Geometry: final body of the model. Coordinates: model frame, mm. Give positions to 0.01 mm unless a question says otherwise; leave off trailing zeros. Write each loop counter-clockwise with the first axis right and the second up, starting at its lowest first coordinate (ties: lowest second). Pieces come first, ordered by that corner, then holes.
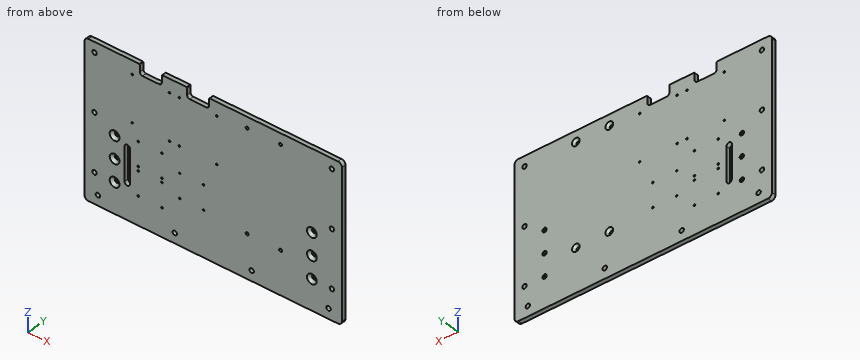
```python
from build123d import *

# Parameters (mm, degrees)
SKETCH1_W                                       = 385
SKETCH1_H                                       = 200
BOSS_EXTRUDE1_DEPTH                             = 6.35
M6_CLEARANCE_HOLE1_D                            = 6.6
CSK_FOR_M6_FLAT_HEAD_MACHINE_SCREW1_AT_2_COUNT  = 2
CSK_FOR_M6_FLAT_HEAD_MACHINE_SCREW1_AT_2_PITCH  = 33
CSK_FOR_M6_FLAT_HEAD_MACHINE_SCREW1_AT_3_COUNT  = 2
CSK_FOR_M6_FLAT_HEAD_MACHINE_SCREW1_AT_3_PITCH  = 66
CSK_FOR_M6_FLAT_HEAD_MACHINE_SCREW1_AT_4_COUNT  = 2
CSK_FOR_M6_FLAT_HEAD_MACHINE_SCREW1_AT_4_PITCH  = 295
CSK_FOR_M6_FLAT_HEAD_MACHINE_SCREW1_AT_5_COUNT  = 2
CSK_FOR_M6_FLAT_HEAD_MACHINE_SCREW1_AT_5_PITCH  = 302.292904316
CSK_FOR_M6_FLAT_HEAD_MACHINE_SCREW1_AT_6_COUNT  = 2
CSK_FOR_M6_FLAT_HEAD_MACHINE_SCREW1_AT_6_PITCH  = 296.840024255
M3X0_5_TAPPED_HOLE1_D                           = 2.5
M3X0_5_TAPPED_HOLE1_DEPTH                       = 7.5
M3X0_5_TAPPED_HOLE1_TIP                         = 0.751075774
CSK_FOR_M4_FLAT_HEAD_MACHINE_SCREW1_D           = 4.5
CSK_FOR_M4_FLAT_HEAD_MACHINE_SCREW1_CSINK_D     = 11.4
CSK_FOR_M4_FLAT_HEAD_MACHINE_SCREW1_CSINK_ANGLE = 90
M3X0_5_TAPPED_HOLE2_D                           = 2.5
CUT_EXTRUDE1_DEPTH                              = 7.35
CUT_EXTRUDE2_DEPTH                              = 7.35
SKETCH18_W                                      = 33
SKETCH18_H                                      = 11
CUT_EXTRUDE3_DEPTH                              = 7.35
FILLET2_R                                       = 1
SKETCH19_W                                      = 385
SKETCH19_H                                      = 6.35
BOSS_EXTRUDE2_DEPTH                             = 30
M6_CLEARANCE_HOLE2_D                            = 6.6
FILLET3_R                                       = 6


with BuildPart() as part:
    # Sketch1 → Boss-Extrude1 (new body)
    with BuildSketch(Plane(origin=(0, 0, 0), x_dir=(1, 0, 0), z_dir=(0, 1, 0))):
        Rectangle(SKETCH1_W, SKETCH1_H)
    extrude(amount=BOSS_EXTRUDE1_DEPTH)

    # M6 Clearance Hole1 (through all)
    with Locations(Plane(origin=(0, 6.35, 0), x_dir=(1, 0, 0), z_dir=(0, 1, 0))):
        with Locations((-177.5, 85), (-177.5, 0), (-177.5, -85)):
            m6_clearance_hole1 = Hole(M6_CLEARANCE_HOLE1_D / 2)

    # Mirror1: M6 Clearance Hole1 across plane
    add(m6_clearance_hole1.mirror(Plane(origin=(0, 0, 0), x_dir=(0, 0, 1), z_dir=(1, 0, 0))), mode=Mode.SUBTRACT)

    # Sketch8 → CSK for M6 Flat Head Machine Screw1 (revolve, cut)
    with BuildSketch(Plane(origin=(147.5, 0, -85), x_dir=(0, 0, -1), z_dir=(1, 0, 0))):
        Polygon((0, 0), (0, 6.35), (3.2, 6.35), (3.2, 4.1), (7.3, 0), align=None)
    csk_for_m6_flat_head_machine_screw1 = revolve(axis=Axis((147.5, -6.35, -85), (0, 1, 0)), mode=Mode.SUBTRACT)

    # CSK for M6 Flat Head Machine Screw1 at 2: CSK for M6 Flat Head Machine Screw1 ×2
    with Locations(*[(0, 0, i * CSK_FOR_M6_FLAT_HEAD_MACHINE_SCREW1_AT_2_PITCH) for i in range(1, CSK_FOR_M6_FLAT_HEAD_MACHINE_SCREW1_AT_2_COUNT)]):
        add(csk_for_m6_flat_head_machine_screw1, mode=Mode.SUBTRACT)

    # CSK for M6 Flat Head Machine Screw1 at 3: CSK for M6 Flat Head Machine Screw1 ×2
    with Locations(*[(0, 0, i * CSK_FOR_M6_FLAT_HEAD_MACHINE_SCREW1_AT_3_PITCH) for i in range(1, CSK_FOR_M6_FLAT_HEAD_MACHINE_SCREW1_AT_3_COUNT)]):
        add(csk_for_m6_flat_head_machine_screw1, mode=Mode.SUBTRACT)

    # CSK for M6 Flat Head Machine Screw1 at 4: CSK for M6 Flat Head Machine Screw1 ×2
    with Locations(*[(-i * CSK_FOR_M6_FLAT_HEAD_MACHINE_SCREW1_AT_4_PITCH, 0, 0) for i in range(1, CSK_FOR_M6_FLAT_HEAD_MACHINE_SCREW1_AT_4_COUNT)]):
        add(csk_for_m6_flat_head_machine_screw1, mode=Mode.SUBTRACT)

    # CSK for M6 Flat Head Machine Screw1 at 5: CSK for M6 Flat Head Machine Screw1 ×2
    with Locations(*[Vector(-0.975874709, 0, 0.218331291) * (i * CSK_FOR_M6_FLAT_HEAD_MACHINE_SCREW1_AT_5_PITCH) for i in range(1, CSK_FOR_M6_FLAT_HEAD_MACHINE_SCREW1_AT_5_COUNT)]):
        add(csk_for_m6_flat_head_machine_screw1, mode=Mode.SUBTRACT)

    # CSK for M6 Flat Head Machine Screw1 at 6: CSK for M6 Flat Head Machine Screw1 ×2
    with Locations(*[Vector(-0.993801293, 0, 0.111170992) * (i * CSK_FOR_M6_FLAT_HEAD_MACHINE_SCREW1_AT_6_PITCH) for i in range(1, CSK_FOR_M6_FLAT_HEAD_MACHINE_SCREW1_AT_6_COUNT)]):
        add(csk_for_m6_flat_head_machine_screw1, mode=Mode.SUBTRACT)

    # M3x0.5 Tapped Hole1
    with Locations(Plane(origin=(0, 0, 0), x_dir=(-1, 0, 0), z_dir=(0, -1, 0))):
        with Locations((-5.317429377, -80), (50.562570623, -80), (65.432985675, -80), (121.312985675, -80), (121.312985675, -11.42), (65.432985675, -11.42), (50.562570623, -11.42), (-5.317429377, -11.42), (76.646256291, 52.44), (76.646256291, 88), (112.206256291, 52.44), (112.206256291, 88), (76.646256291, 46.44), (112.206256291, 46.44), (112.206256291, 10.88), (76.646256291, 10.88)):
            Hole(M3X0_5_TAPPED_HOLE1_D / 2, depth=M3X0_5_TAPPED_HOLE1_DEPTH)
            with Locations((0, 0, -(M3X0_5_TAPPED_HOLE1_DEPTH + M3X0_5_TAPPED_HOLE1_TIP / 2))):  # 118° drill point
                Cone(0, M3X0_5_TAPPED_HOLE1_D / 2, M3X0_5_TAPPED_HOLE1_TIP, mode=Mode.SUBTRACT)

    # CSK for M4 Flat Head Machine Screw1 (through all)
    with Locations(Plane(origin=(0, 6.35, 0), x_dir=(1, 0, 0), z_dir=(0, 1, 0))):
        with Locations((50.75, -84), (100.75, -84), (50.75, 66), (100.75, 66)):
            CounterSinkHole(CSK_FOR_M4_FLAT_HEAD_MACHINE_SCREW1_D / 2, CSK_FOR_M4_FLAT_HEAD_MACHINE_SCREW1_CSINK_D / 2, counter_sink_angle=CSK_FOR_M4_FLAT_HEAD_MACHINE_SCREW1_CSINK_ANGLE)

    # M3x0.5 Tapped Hole2 (through all)
    with Locations(Plane(origin=(0, 0, 0), x_dir=(-1, 0, 0), z_dir=(0, -1, 0))):
        with Locations((14.506651869, 62.535124228), (50.066651869, 62.535124228), (50.066651869, 26.975124228), (14.506651869, 26.975124228)):
            Hole(M3X0_5_TAPPED_HOLE2_D / 2)

    # Sketch16 → Cut-Extrude1 (cut, through all)
    with BuildSketch(Plane.XZ):
        with BuildLine():
            Line((-124.5, -27), (-124.5, -77))
            ThreePointArc((-124.5, -77), (-128.5, -81), (-132.5, -77))
            Line((-132.5, -77), (-132.5, -27))
            ThreePointArc((-132.5, -27), (-128.5, -23), (-124.5, -27))
        make_face()
    extrude(amount=-CUT_EXTRUDE1_DEPTH, mode=Mode.SUBTRACT)

    # Sketch17 → Cut-Extrude2 (cut, through all)
    with BuildSketch(Plane.XZ):
        with BuildLine():
            Line((-105.872985675, 93), (-80.872985675, 93))
            ThreePointArc((-80.872985675, 93), (-76.872985675, 89), (-80.872985675, 85))
            Line((-80.872985675, 85), (-105.872985675, 85))
            ThreePointArc((-105.872985675, 85), (-109.872985675, 89), (-105.872985675, 93))
        make_face()
        with BuildLine():
            Line((-35.122570623, 93), (-10.122570623, 93))
            ThreePointArc((-10.122570623, 93), (-6.122570623, 89), (-10.122570623, 85))
            Line((-10.122570623, 85), (-35.122570623, 85))
            ThreePointArc((-35.122570623, 85), (-39.122570623, 89), (-35.122570623, 93))
        make_face()
    extrude(amount=-CUT_EXTRUDE2_DEPTH, mode=Mode.SUBTRACT)

    # Sketch18 → Cut-Extrude3 (cut, through all)
    with BuildSketch(Plane.XZ):
        with Locations((-22.622570623, 94.5)):
            Rectangle(SKETCH18_W, SKETCH18_H)
        with Locations((-93.372985675, 94.5)):
            Rectangle(SKETCH18_W, SKETCH18_H)
    extrude(amount=-CUT_EXTRUDE3_DEPTH, mode=Mode.SUBTRACT)

    # Fillet2
    fillet2_edges = [part.edges().sort_by_distance(p)[0] for p in [
        (-6.122570623, 3.175, 100),
        (-39.122570623, 3.175, 100),
        (-76.872985675, 3.175, 100),
        (-109.872985675, 3.175, 100),
    ]]
    fillet(fillet2_edges, radius=FILLET2_R)

    # Sketch19 → Boss-Extrude2 (add)
    with BuildSketch(Plane(origin=(0, 0, -100), x_dir=(-1, 0, 0), z_dir=(0, 0, -1))):
        with Locations((0, 3.175)):
            Rectangle(SKETCH19_W, SKETCH19_H)
    extrude(amount=BOSS_EXTRUDE2_DEPTH)

    # M6 Clearance Hole2 (through all)
    with Locations(Plane(origin=(0, 0, 0), x_dir=(-1, 0, 0), z_dir=(0, -1, 0))):
        with Locations((-172.5, 115), (172.5, 115), (-57.5, 115), (57.5, 115)):
            Hole(M6_CLEARANCE_HOLE2_D / 2)

    # Fillet3
    fillet3_edges = [part.edges().sort_by_distance(p)[0] for p in [
        (192.5, 3.175, -130),
        (-192.5, 3.175, -130),
        (192.5, 3.175, 100),
        (-192.5, 3.175, 100),
    ]]
    fillet(fillet3_edges, radius=FILLET3_R)


solid = part.part
```
Item 1: Pin query (flat end, axial travel): pin 1 Ø1.5 at (x, z) = (-14.51, -26.98) entering from -Y. Return the tip coordinate at first contact, or that it passes through.
Found:
pin 1: passes through
Item 2: Section A-A, the plane x = -100.5. Return the cut outline in (y, z).
Found:
outline: (0, -130) - (6.35, -130) - (6.35, 85) - (0, 85) - close
Item 3: Line query: L1, parallel to Z at x = 147.5, y = 4.75; L2, parallel to X at y = 1.65, z = -66; L3, parallel to X at y = 3.25, z = -46. Output: solid intervals per line, ascending.
Found:
L1: z = -130 to -88.2, -81.8 to -55.2, -48.8 to -22.2, -15.8 to 100
L2: x = -192.5 to -132.5, -124.5 to 48.5, 53 to 98.5, 103 to 192.5
L3: x = -192.5 to -132.5, -124.5 to -113.38, -111.04 to -77.82, -75.48 to 192.5
